Build history of the part. All positions in model axes, mm. A direction names the side the tool comes from. Round coordinates to 2 decimals unless told otherwise and drop trailing zeros. Write each loop counter-clockwise with the first axis right and the second up, starting at its lowest first coordinate (ties: lowest second). Pieces come first, ordered by that corner, then holes. Notation, with made-up numbers: (76.5, 75.25) -> (94.5, 75.25) arc R19 ccw to (94.5, 104.25) -> close; hole circle Ø7 at (32, 37.25). An arc over 180 degrees is marked (long way). Answer as CSV lines item,"result".
Autodesk Inventor part; units mm, degrees
ref_plane "YZ Plane" through (0, 0, 0) normal (1, 0, 0) x (0, 1, 0)
ref_plane "XZ Plane" through (0, 0, 0) normal (0, 1, 0) x (-1, 0, 0)
ref_plane "XY Plane" through (0, 0, 0) normal (0, 0, 1) x (1, 0, 0)
sketch "Sketch1" plane through (0, 0, 0) normal (0, 0, 1) x (1, 0, 0)
  line L0 (0, 0) -> (15, 0)
  line L1 (15, 0) -> (15, 10)
  line L2 (15, 10) -> (0, 10)
  line L3 (0, 10) -> (0, 0)
  line L4 (1, 9) -> (14, 9)
  line L5 (14, 9) -> (14, 1)
  line L6 (14, 1) -> (1, 1)
  line L7 (1, 1) -> (1, 9)
  dimension "d0" = 15
  dimension "d1" = 10
  dimension "d2" = 13
  dimension "d3" = 8
  dimension "d4" = 1
  dimension "d5" = 1
extrude "Extrusion1" add sketch "Sketch1" along normal blind 90
sketch "Sketch2" plane through (0, 10, 0) normal (0, 1, 0) x (1, 0, 0)
  line L0 (15, 0) -> (0, 0)
  line L1 (0, 0) -> (0, -90)
  line L2 (15, -90) -> (0, -90)
  line L3 (15, 0) -> (15, -90)
  circle A0 centre (7.5, -9.5) radius 1.5
  circle A1 centre (7.5, -74.5) radius 1.5
  circle A2 centre (7.5, -19.5) radius 1.5
  circle A3 centre (7.5, -64.5) radius 1.5
  circle A4 centre (7.5, -54.5) radius 1.5
  circle A5 centre (7.5, -38.5) radius 1.5
  dimension "d8" = 3
  dimension "d9" = 3
  dimension "d10" = 7.5
  dimension "d11" = 7.5
  dimension "d12" = 9.5
  dimension "d13" = 15.5
  dimension "d24" = 3
  dimension "d25" = 3
  dimension "d26" = 3
  dimension "d27" = 3
  dimension "d28" = 7.5
  dimension "d29" = 7.5
  dimension "d30" = 7.5
  dimension "d31" = 7.5
  dimension "d32" = 10
  dimension "d33" = 10
  dimension "d34" = 10
  dimension "d35" = 16
extrude "Extrusion2" cut sketch "Sketch2" against normal up to surface (10 mm away) contours A0 | A1 | A2 | A3 | A4 | A5
sketch "Sketch3" plane through (15, 0, 0) normal (1, 0, 0) x (0, 0, -1)
  line L0 (0, 0) -> (0, 10)
  line L1 (0, 10) -> (-90, 10)
  line L2 (-90, 0) -> (-90, 10)
  line L3 (0, 0) -> (-90, 0)
  circle A0 centre (-9, 5) radius 1.5
  circle A1 centre (-85, 5) radius 1.5
  dimension "d16" = 3
  dimension "d17" = 5
  dimension "d18" = 9
  dimension "d21" = 3
  dimension "d22" = 5
  dimension "d23" = 5
extrude "Extrusion3" [suppressed]
properties part number "profile4" material "Aluminum 6061, Welded"
1. Drop flat-ended pins along their axis: pin 1 Ø3.5 at (x, z) = (7.5, 38.5) entering from +Y; pin 2 Ø1 at (x, y) = (7, 7) entering from +Z. Give the stop position or say it passes through.
Results found:
pin 1,"stops at y = 10"
pin 2,"passes through"
2. Mould opens along X. For faces 3 (the flat face through (15, 5, 44)), 4 (the cylindrical face through (7.305, 9.507, 63.013)), 5 (the flat face through (7.4, 0.6, 0)) say: +X half, -X half, draft (parallel to the pull), parting line (faces both ways), or undercut.
Results found:
face 3,"+X half"
face 4,"undercut"
face 5,"draft"
3. Which spindle directions (+Z, -Z, +X, -X, +Y, -Y) get a long thin tool onto all of the face, cutting with end or side? Do faces 1 (the cylindrical face through (6.3, 0.5, 10.4)), 2 (the flat face through (14, 5, 44)). Say none if no direction does.
Results found:
face 1,"+Y, -Y"
face 2,"+Z, -Z"
4. Cut at B-B, the plane z = 9.5. Write the cut outline in (x, y).
Results found:
outline,"(0, 0) -> (6, 0) -> (6, 1) -> (1, 1) -> (1, 9) -> (6, 9) -> (6, 10) -> (0, 10) -> close; (9, 0) -> (15, 0) -> (15, 10) -> (9, 10) -> (9, 9) -> (14, 9) -> (14, 1) -> (9, 1) -> close"
5. Cut at D-D, the plane x = 8. Count the separate pieces of the cut face and the enclosed holes in it, then the cut area to 3 significant figures.
Results found:
separate pieces,"14"
enclosed holes,"0"
area,"146 mm2"
6. Probe line 1 along X through (y, z) = (4, 37.5); line 2 along Y through (x, z) = (12, 55); line 3 along X through (y, z) = (0.75, 19.5). List the from-to ranges inside material, lowest first.
Results found:
line 1,"x = 0 to 1, 14 to 15"
line 2,"y = 0 to 1, 9 to 10"
line 3,"x = 0 to 6, 9 to 15"
7. Cut at C-C, the plane z = 26. Write the cut outline in (x, y).
Results found:
outline,"(0, 0) -> (15, 0) -> (15, 10) -> (0, 10) -> close; hole (1, 1) -> (14, 1) -> (14, 9) -> (1, 9) -> close"
8. Cut at A-A, the plane y = 3. Write the cut outline in (x, z), then the cut area to 3 significant figures.
Results found:
outline,"(0, 0) -> (1, 0) -> (1, 90) -> (0, 90) -> close; (14, 0) -> (15, 0) -> (15, 90) -> (14, 90) -> close"
area,"180 mm2"
